Part model, mm, in its own coordinate system. Face numbers are marked on the shaded views. A direction names the side the tool comes from. Give positions to 0.01 mm unless a question says otherwise; leave off trailing zeros. Order: outer loops, then holes, each group sorted by start corner. A loop starts at its lowest first (then second) coordinate and runs counter-clockwise, first axis right, second up. Notation, with made-up numbers: M -8.75,-6 L 32.25,-6 A23 ccw 32.25,25 Z; hole C 77.5,89.25 d8. An arc over 180 degrees is marked long. One line per question, with ' | ' between items.
```python
from build123d import *

# Parameters (mm, degrees)
PAD002_DEPTH    = 12
SKETCH017_R     = 2.5
POCKET014_DEPTH = 10
POCKET015_DEPTH = 1
SKETCH019_W     = 8
SKETCH019_H     = 8.3
POCKET016_DEPTH = 5
PAD003_DEPTH    = 2.5


with BuildPart() as part:
    # Sketch016 → Pad002 (new body)
    with BuildSketch(Plane.XY):
        with BuildLine():
            ThreePointArc((0, 0), (0.0125001507, 3.6000868045), (0.05, 7.2))
            Line((0.05, 7.2), (0.75, 22.55))
            add(Edge.make_bspline(
                [(0.75, 22.55), (0.790433, 24.50555), (2.8995135699, 28.3383927733), (10.6468681476, 35.231617337), (14.5053016695, 34.8194742751), (20.1, 35.5)],
                knots=[0, 0, 0, 0, 0.3333333333, 0.6666666667, 1, 1, 1, 1], degree=3))
            Line((20.1, 35.5), (64.2, 35.5))
            add(Edge.make_bspline(
                [(92, 0), (92.391037, 11.810127), (88.126587, 35.076866), (64.2, 35.5)],
                knots=[0, 0, 0, 0, 1, 1, 1, 1], degree=3))
            Line((92, 0), (0, 0))
        make_face()
    extrude(amount=PAD002_DEPTH)

    # Sketch017 (on Face8 of Pad002) → Pocket014 (cut)
    with BuildSketch(Plane.XY.offset(12)):
        with Locations((17, 25)):
            Circle(SKETCH017_R)
        with BuildLine():
            ThreePointArc((84.5, 0), (82, 2.5), (79.5, 0))
            Line((79.5, 0), (84.5, 0))
        make_face()
        with BuildLine():
            Line((2, 0), (2.5758571429, 18.6857169977))
            ThreePointArc((7.6817324497, 29.5040514173), (4.0036624605, 24.625907301), (2.5758571429, 18.6857169977))
            ThreePointArc((11, 28), (9.8256709089, 29.8216112511), (7.6817324497, 29.5040514173))
            Line((11, 25), (11, 28))
            ThreePointArc((11, 25), (17, 19), (23, 25))
            Line((23, 25), (23, 31.5))
            ThreePointArc((25, 33.5), (23.5857864376, 32.9142135624), (23, 31.5))
            Line((28, 33.5), (25, 33.5))
            ThreePointArc((30, 31.5), (29.4142135624, 32.9142135624), (28, 33.5))
            Line((30, 12), (30, 31.5))
            ThreePointArc((30, 12), (30.5857864376, 10.5857864376), (32, 10))
            Line((34, 10), (32, 10))
            ThreePointArc((34, 10), (35.4142135624, 10.5857864376), (36, 12))
            Line((36, 31.5), (36, 12))
            ThreePointArc((38, 33.5), (36.5857864376, 32.9142135624), (36, 31.5))
            Line((45.2, 33.5), (38, 33.5))
            ThreePointArc((47.2, 31.5), (46.6142135624, 32.9142135624), (45.2, 33.5))
            Line((47.2, 12), (47.2, 31.5))
            ThreePointArc((47.2, 12), (47.7857864376, 10.5857864376), (49.2, 10))
            Line((51.2, 10), (49.2, 10))
            ThreePointArc((51.2, 10), (52.6142135624, 10.5857864376), (53.2, 12))
            Line((53.2, 31.4999999999), (53.2, 12))
            ThreePointArc((55.2, 33.4999999999), (53.7857864376, 32.9142135623), (53.2, 31.4999999999))
            Line((55.2, 33.5), (64.2, 33.5))
            ThreePointArc((87.491325765, 7.8139309331), (81.5019467421, 25.7859071373), (64.2, 33.5))
            ThreePointArc((85.5, 6), (86.8468225322, 6.521463877), (87.491325765, 7.8139309331))
            Line((82, 6), (85.5, 6))
            ThreePointArc((82, 6), (77.7573593129, 4.2426406871), (76, 0))
            Line((22, 0), (76, 0))
            Line((22, 1), (22, 0))
            Line((16, 1), (22, 1))
            Line((16, 0), (16, 1))
            Line((2, 0), (16, 0))
        make_face()
    extrude(amount=-POCKET014_DEPTH, mode=Mode.SUBTRACT)

    # Sketch018 (on Face3 of Pocket014) → Pocket015 (cut)
    with BuildSketch(Plane.XZ):
        Polygon((22, 12), (22, 4), (18, 10), (16, 10), (16, 12), align=None)
    extrude(amount=-POCKET015_DEPTH, mode=Mode.SUBTRACT)

    # Sketch019 → Pocket016 (cut)
    with BuildSketch(Plane.YZ):
        with Locations((4, 6.15)):
            Rectangle(SKETCH019_W, SKETCH019_H)
    extrude(amount=POCKET016_DEPTH, mode=Mode.SUBTRACT)

    # Sketch022 (on Face8 of Pocket016) → Pad003 (join)
    with BuildSketch(Plane.XY.offset(12)):
        with BuildLine():
            ThreePointArc((34, 10), (35.4142135624, 10.5857864376), (36, 12))
            Line((36, 12), (36, 14))
            ThreePointArc((36, 14), (35.4142135624, 15.4142135624), (34, 16))
            Line((32, 16), (34, 16))
            ThreePointArc((32, 16), (30.5857864376, 15.4142135624), (30, 14))
            Line((30, 12), (30, 14))
            ThreePointArc((30, 12), (30.5857864376, 10.5857864376), (32, 10))
            Line((32, 10), (34, 10))
        make_face()
        with BuildLine():
            ThreePointArc((47.2, 12), (47.7857864376, 10.5857864376), (49.2, 10))
            Line((49.2, 10), (51.2, 10))
            ThreePointArc((51.2, 10), (52.6142135624, 10.5857864376), (53.2, 12))
            Line((53.2, 12), (53.2, 14))
            ThreePointArc((53.2, 14), (52.6142135624, 15.4142135624), (51.2, 16))
            Line((49.2, 16), (51.2, 16))
            ThreePointArc((49.2, 16), (47.7857864376, 15.4142135624), (47.2, 14))
            Line((47.2, 12), (47.2, 14))
        make_face()
    extrude(amount=PAD003_DEPTH)

    # Mirrored001: part across XZ


with BuildPart() as part_1:
    add(part.part)
    add(part.part.mirror(Plane.XZ))


with BuildPart() as part_2:
    # Body002 placement: moved
    add(part_1.part.moved(Location((0, 0, -12))))


solid = part_2.part
```
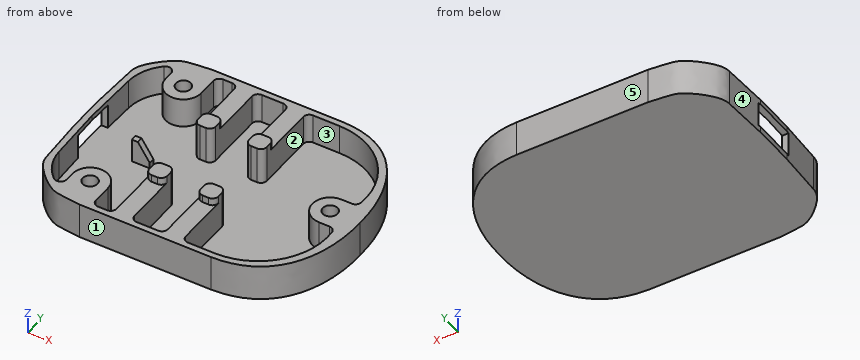
1. Probe L1, parallel to Y at x = 60.5, z = -7; L2, parallel to X at y = -31, z = -1; L3, parallel to Y at x = 17, z = -4.25. List the from-to ranges inside material, lowest first. Write a range as from..to.
Worked out:
L1: y = -35.5..-33.5, 33.5..35.5 | L2: x = 6.08..23, 30..36, 47.2..53.2, 74.64..79.34 | L3: y = -35.17..-27.5, -22.5..-19, -1..1, 19..22.5, 27.5..35.17
2. Slice it at A-A on x = 60.5. Give the cut face in (y, z).
Worked out:
outline: M -35.5,-12 L 35.5,-12 L 35.5,0 L 33.5,0 L 33.5,-10 L -33.5,-10 L -33.5,0 L -35.5,0 Z
3. Slice it at B-B on z = -3.5. Give the number of separate pieces and of enclosed holes in the cut face, then the cut area to 3 significant figures.
Worked out:
separate pieces: 2 | enclosed holes: 3 | area: 1,570 mm2
4. Tool access for the marked faces 1 and 2: list every direction of +Z, -Z, +X, -X, +Y, -Y with a clear straight run to the whole face (end or side of a thin tool).
Worked out:
face 1: +Z, -Z, +X, -X, -Y | face 2: +Z
5. Mould opens along X. For the marked faces 3, 4 and 5 say: released by +X, released by -X, zero draft, split by the parting line, or undercut.
Worked out:
face 3: undercut | face 4: released by -X | face 5: zero draft
6. Drop flat-ended pins along their axis: pin 1 (2.5 mm diameter, centred on x = 1.5, z = -7.5, fed in from +Y); pin 2 (5 mm diameter, centred on y = 29.5, z = -4.5, fed in from +X); pin 3 (1 mm diameter, centred on y = 11, z = -6, fed in from +X); pin 4 (3 mm diameter, centred on y = -3, z = -2, fed in from +X). Give the stop position or say it passes through.
Worked out:
pin 1: stops at y = 27.4 | pin 2: stops at x = 83.79 | pin 3: stops at x = 91.18 | pin 4: stops at x = 92.02
